Source: CAD feature listing. Evaluate the final solid. Frame: model axes, mm. Face numbers are marked on the shaded views. A direction names the side the tool comes from. Give positions to 0.01 mm unless a question says otherwise; leave off trailing zeros. Loops run counter-clockwise (first coordinate to the right, second up) from the corner with the lowest first, then second, coordinate; pieces in that order, holes last.
```python
from build123d import *

# Parameters (mm, degrees)
ESBO_O2_W             = 152
ESBO_O2_H             = 115
BASE_DEPTH            = 4.5
ESBO_O3_W             = 152
ESBO_O3_H             = 115
ESBO_O3_W_2           = 146.4
ESBO_O3_H_2           = 109.4
PAREDES_DEPTH         = 20
CHANFRO_DA_BASE_SIZE  = 3
FILETE7_R             = 3
FILETE8_R             = 3
FILETE10_R            = 2
FILETE12_R            = 2
CHANFRO8_SIZE         = 3
CHANFRO9_SIZE         = 3
CHANFRO14_SIZE        = 5
CHANFRO17_SIZE        = 5
CORTE_EXTRUS_O4_DEPTH = 10


with BuildPart() as part:
    # Esboço2 → Base (new body)
    with BuildSketch(Plane(origin=(0, 0, 0), x_dir=(1, 0, 0), z_dir=(0, 1, 0))):
        Rectangle(ESBO_O2_W, ESBO_O2_H)
    extrude(amount=BASE_DEPTH)

    # Esboço3 → Paredes (add)
    with BuildSketch(Plane(origin=(0, 4.5, 0), x_dir=(1, 0, 0), z_dir=(0, 1, 0))):
        Rectangle(ESBO_O3_W, ESBO_O3_H)
        Rectangle(ESBO_O3_W_2, ESBO_O3_H_2, mode=Mode.SUBTRACT)
    extrude(amount=PAREDES_DEPTH)

    # Chanfro da Base
    chanfro_da_base_edges = [part.edges().sort_by_distance(p)[0] for p in [
        (0, 4.5, -54.7),
        (-73.2, 4.5, 0),
        (0, 4.5, 54.7),
        (73.2, 4.5, 0),
    ]]
    chamfer(chanfro_da_base_edges, length=CHANFRO_DA_BASE_SIZE)

    # Filete7
    filete7_edges = [part.edges().sort_by_distance(p)[0] for p in [
        (-76, 12.25, 57.5),
    ]]
    fillet(filete7_edges, radius=FILETE7_R)

    # Filete8
    filete8_edges = [part.edges().sort_by_distance(p)[0] for p in [
        (76, 12.25, 57.5),
    ]]
    fillet(filete8_edges, radius=FILETE8_R)

    # Filete10
    filete10_edges = [part.edges().sort_by_distance(p)[0] for p in [
        (-76, 12.25, -57.5),
    ]]
    fillet(filete10_edges, radius=FILETE10_R)

    # Filete12
    filete12_edges = [part.edges().sort_by_distance(p)[0] for p in [
        (76, 12.25, -57.5),
    ]]
    fillet(filete12_edges, radius=FILETE12_R)

    # Chanfro8
    chanfro8_edges = [part.edges().sort_by_distance(p)[0] for p in [
        (-73.2, 16, 54.7),
    ]]
    chamfer(chanfro8_edges, length=CHANFRO8_SIZE)

    # Chanfro9
    chanfro9_edges = [part.edges().sort_by_distance(p)[0] for p in [
        (73.2, 16, 54.7),
    ]]
    chamfer(chanfro9_edges, length=CHANFRO9_SIZE)

    # Chanfro14
    chanfro14_edges = [part.edges().sort_by_distance(p)[0] for p in [
        (-73.2, 16, -54.7),
    ]]
    chamfer(chanfro14_edges, length=CHANFRO14_SIZE)

    # Chanfro17
    chanfro17_edges = [part.edges().sort_by_distance(p)[0] for p in [
        (73.2, 16, -54.7),
    ]]
    chamfer(chanfro17_edges, length=CHANFRO17_SIZE)

    # Esboço6 → Corte-extrusão4 (cut)
    with BuildSketch(Plane(origin=(0, 0, -57.5), x_dir=(-1, 0, 0), z_dir=(0, 0, -1))):
        with BuildLine():
            Line((16.5, 17.5), (16.5, 14.5))
            ThreePointArc((16.5, 14.5), (17.085786438, 13.085786438), (18.5, 12.5))
            Line((18.5, 12.5), (21.5, 12.5))
            ThreePointArc((21.5, 12.5), (22.914213562, 13.085786438), (23.5, 14.5))
            Line((23.5, 14.5), (23.5, 17.5))
            ThreePointArc((23.5, 17.5), (22.914213562, 18.914213562), (21.5, 19.5))
            Line((21.5, 19.5), (18.5, 19.5))
            ThreePointArc((18.5, 19.5), (17.085786438, 18.914213562), (16.5, 17.5))
        make_face()
        with BuildLine():
            Line((-21.5, 19.5), (-18.5, 19.5))
            ThreePointArc((-18.5, 19.5), (-17.085786438, 18.914213562), (-16.5, 17.5))
            Line((-16.5, 17.5), (-16.5, 14.5))
            ThreePointArc((-16.5, 14.5), (-17.085786438, 13.085786438), (-18.5, 12.5))
            Line((-18.5, 12.5), (-21.5, 12.5))
            ThreePointArc((-21.5, 12.5), (-22.914213562, 13.085786438), (-23.5, 14.5))
            Line((-23.5, 14.5), (-23.5, 17.5))
            ThreePointArc((-23.5, 17.5), (-22.914213562, 18.914213562), (-21.5, 19.5))
        make_face()
        with BuildLine():
            Line((46.5, 17.5), (46.5, 14.5))
            ThreePointArc((46.5, 14.5), (47.085786438, 13.085786438), (48.5, 12.5))
            Line((48.5, 12.5), (51.5, 12.5))
            ThreePointArc((51.5, 12.5), (52.914213562, 13.085786438), (53.5, 14.5))
            Line((53.5, 14.5), (53.5, 17.5))
            ThreePointArc((53.5, 17.5), (52.914213562, 18.914213562), (51.5, 19.5))
            Line((51.5, 19.5), (48.5, 19.5))
            ThreePointArc((48.5, 19.5), (47.085786438, 18.914213562), (46.5, 17.5))
        make_face()
        with BuildLine():
            Line((-51.5, 19.5), (-48.5, 19.5))
            ThreePointArc((-48.5, 19.5), (-47.085786438, 18.914213562), (-46.5, 17.5))
            Line((-46.5, 17.5), (-46.5, 14.5))
            ThreePointArc((-46.5, 14.5), (-47.085786438, 13.085786438), (-48.5, 12.5))
            Line((-48.5, 12.5), (-51.5, 12.5))
            ThreePointArc((-51.5, 12.5), (-52.914213562, 13.085786438), (-53.5, 14.5))
            Line((-53.5, 14.5), (-53.5, 17.5))
            ThreePointArc((-53.5, 17.5), (-52.914213562, 18.914213562), (-51.5, 19.5))
        make_face()
    extrude(amount=-CORTE_EXTRUS_O4_DEPTH, mode=Mode.SUBTRACT)


solid = part.part
```
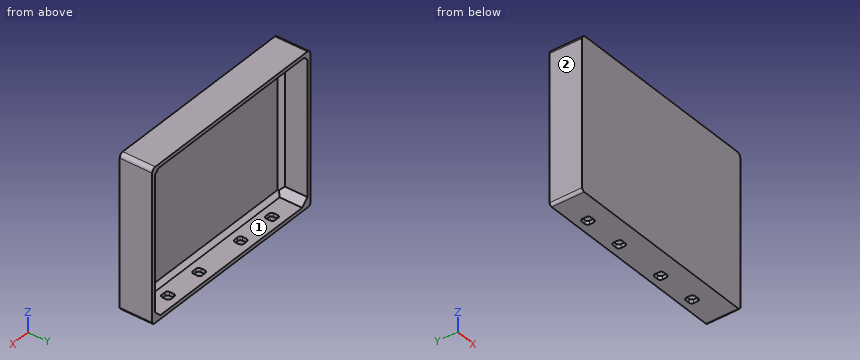
(1) Section B-B, the plane x = -56. Return the cut outline in (y, z).
A:
outline: (0, -57.5) - (24.5, -57.5) - (24.5, -54.7) - (7.5, -54.7) - (4.5, -51.7) - (4.5, 51.7) - (7.5, 54.7) - (24.5, 54.7) - (24.5, 57.5) - (0, 57.5) - close
(2) First-contact query: pin 1 (0.8 mm diameter, centred on y = 16, z = -56.5, fed in from +X); pin 2 (5 mm diameter, centred on x = -22.5, z = -3.5, fed in from +Y); pin 3 (0.8 mm diameter, centred on y = 15.5, z = -56, fed in from -X). Flat tips, straight axial feed; report the tip coordinate or a pass-through.
A:
pin 1: stops at x = 75.91
pin 2: stops at y = 4.5
pin 3: stops at x = -76
(3) Section C-C, the plane z = -6. Return the cut outline in (x, y), then the cut area to 3 significant figures.
A:
outline: (-76, 0) - (76, 0) - (76, 24.5) - (73.2, 24.5) - (73.2, 7.5) - (70.2, 4.5) - (-70.2, 4.5) - (-73.2, 7.5) - (-73.2, 24.5) - (-76, 24.5) - close
area: 805 mm2
(4) Section A-A, the plane y = 22.5. Return the cut outline in (x, z), then the cut area to 3 significant figures.
A:
outline: (-76, -55.5) arc R2 ccw to (-74, -57.5) - (74, -57.5) arc R2 ccw to (76, -55.5) - (76, 54.5) arc R3 ccw to (73, 57.5) - (-73, 57.5) arc R3 ccw to (-76, 54.5) - close; hole (-73.2, -49.7) - (-68.2, -54.7) - (68.2, -54.7) - (73.2, -49.7) - (73.2, 51.7) - (70.2, 54.7) - (-70.2, 54.7) - (-73.2, 51.7) - close
area: 1,490 mm2
(5) Ray query, line 1 along Z through (x, y) = (-61, 20); line 2 along X through (y, z) = (18, -40.5); line 3 along Y through (x, z) = (-51, -25). Return the intervals inside material, ascending.
A:
line 1: z = -57.5 to -54.7, 54.7 to 57.5
line 2: x = -76 to -73.2, 73.2 to 76
line 3: y = 0 to 4.5
(6) Reachability of the marked faces 1 and 2 from +Z, -Z, +X, -X, +Y, -Y: full face, straight path, thin tool, end or side. Return the list, or none.
A:
face 1: +Y
face 2: +Z, -Z, -X, +Y, -Y
